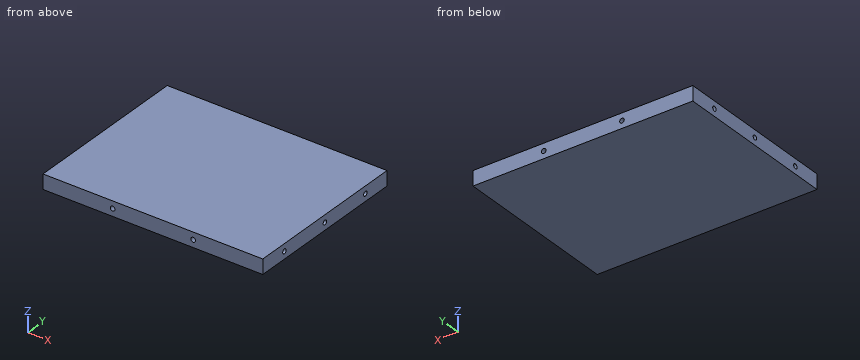
Autodesk Inventor part; units mm, degrees
ref_plane "YZ Plane" through (0, 0, 0) normal (1, 0, 0) x (0, 1, 0)
ref_plane "XZ Plane" through (0, 0, 0) normal (0, 1, 0) x (-1, 0, 0)
ref_plane "XY Plane" through (0, 0, 0) normal (0, 0, 1) x (1, 0, 0)
sketch "Sketch1" plane through (0, 0, 0) normal (0, 0, 1) x (1, 0, 0)
  line L0 (-75, 57.5) -> (75, 57.5)
  line L1 (75, 57.5) -> (75, -57.5)
  line L2 (75, -57.5) -> (-75, -57.5)
  line L3 (-75, -57.5) -> (-75, 57.5)
  line L4 (-75, 57.5) -> (75, -57.5) construction
  line L5 (75, 57.5) -> (-75, -57.5) construction
  point P0 (0, 0)
  dimension "d0" = 150
  dimension "d1" = 115
extrude "Extrusion1" add sketch "Sketch1" along normal mid plane 10
sketch "Sketch2" plane through (75, -57.5, 5) normal (1, 0, 0) x (0, 0, -1)
  line L0 (10, 0) -> (0, 0)
  line L1 (0, 0) -> (0, 115)
  point P0 (5, 57.5)
  point P1 (5, 20)
  point P2 (5, 57.5)
  point P3 (5, 95)
  dimension "d4" = 20
  dimension "d5" = 5
  dimension "d8" = 37.5
hole "Hole1" at (75, -37.5, 0) at (75, 0, 0) at (75, 37.5, 0) direction (-1, 0, 0) diameter 3.175 depth 5
sketch "Sketch3" plane through (-75, 57.5, 5) normal (0, 1, 0) x (1, 0, 0)
  line L0 (150, 10) -> (150, 0)
  line L1 (0, 10) -> (150, 10)
  point P0 (75, 5)
  point P1 (101.6667, 5)
  point P2 (48.3333, 5)
  dimension "d21" = 5
  dimension "d24" = 53.3333
  dimension "d69" = 26.6667
hole "Hole2" at (26.6667, 57.5, 0) at (-26.6667, 57.5, 0) direction (0, -1, 0) diameter 3.175 depth 5
sketch "Sketch4" plane through (-75, -57.5, 5) normal (0, -1, 0) x (1, 0, 0)
  line L0 (150, -10) -> (150, 0)
  line L1 (0, 0) -> (150, 0)
  point P0 (75, -5)
  point P1 (102.5, -5)
  point P2 (47.5, -5)
  dimension "d37" = 5
  dimension "d40" = 55
  dimension "d68" = 27.5
hole "Hole3" at (27.5, -57.5, 0) at (-27.5, -57.5, 0) direction (0, 1, 0) diameter 3.175 depth 5
sketch "Sketch5" plane through (-75, -57.5, 5) normal (-1, 0, 0) x (0, 0, 1)
  line L0 (0, 0) -> (-10, 0)
  line L1 (-10, 0) -> (-10, 115)
  point P0 (-5, 57.5)
  point P1 (-5, 20)
  point P2 (-5, 57.5)
  point P3 (-5, 95)
  dimension "d52" = 20
  dimension "d53" = 5
  dimension "d56" = 37.5
hole "Hole4" at (-75, -37.5, 0) at (-75, 0, 0) at (-75, 37.5, 0) direction (1, 0, 0) diameter 3.175 depth 5
properties part number "front"
Work out the finished part from the listing and answer in its coordinate system (mm). Round coordinates to 2 decimals unless told otherwise and drop trailing zeros. Write each loop counter-clockwise with the first axis right and the second up, starting at its lowest first coordinate (ties: lowest second). Pieces come first, ordered by that corner, then holes.
1) Straight lines are drawn through the part: line 1 (Y direction, x = 73.9, z = 0); line 2 (X direction, y = 56.25, z = 0); line 3 (Z direction, x = 71.55, y = -37.5). For each, find the intervals that lie inside material, in ascending order.
2) A cutting plane is placed at A-A (y = 37.5). Give the vertices of the cut face in (x, z).
3) Given pin 1 Ø2.5 at (y, z) = (0, 0) entering from +X; pin 2 Ø1.6 at (x, z) = (-28, -0.5) entering from -Y; pin 3 Ø1.9 at (y, z) = (37.5, 0) entering from -X, each flat-ended and moving along its own axis, determine where each tip first touches the part or whether it passes through.
Completed:
1. line 1: y = -57.5 to -39.09, -35.91 to -1.59, 1.59 to 35.91, 39.09 to 57.5
1. line 2: x = -75 to -28.25, -25.08 to 25.08, 28.25 to 75
1. line 3: z = -5 to -1.59, 1.59 to 5
2. outline: (-75, -5) - (75, -5) - (75, -1.59) - (70, -1.59) - (70, 1.59) - (75, 1.59) - (75, 5) - (-75, 5) - (-75, 1.59) - (-70, 1.59) - (-70, -1.59) - (-75, -1.59) - close
3. pin 1: stops at x = 70
3. pin 2: stops at y = -52.5
3. pin 3: stops at x = -70
